from build123d import *

# Parameters (mm, degrees)
SKETCH1_W           = 22.8
SKETCH1_H           = 55
SKETCH1_W_2         = 25
SKETCH1_H_2         = 6
SKETCH1_W_3         = 7.1
SKETCH1_H_3         = 8.35
SKETCH2_R           = 6.05
BOSS_EXTRUDE1_DEPTH = 5.6
SKETCH2_3_W         = 10.7
SKETCH2_3_H         = 16.7
BOSS_EXTRUDE2_DEPTH = 13.8


with BuildPart() as part:
    # Sketch1 → Revolve1 (revolve)
    with BuildSketch(Plane.XY, mode=Mode.PRIVATE) as revolve1_sk:
        with BuildLine():
            Line((-24.6, 0), (0, 0))
            Line((0, 0), (0, 100))
            ThreePointArc((0, 100), (-13.097327972, 97.679363123), (-24.6, 91))
            Line((-24.6, 91), (-24.6, 68.856406461))
            Line((-24.6, 68.856406461), (-24.6, 0))
        make_face()
        with BuildLine():
            Line((0, 100), (0, 0))
            Line((0, 0), (24.6, 0))
            Line((24.6, 0), (24.6, 68.856406461))
            Line((24.6, 68.856406461), (24.6, 91))
            ThreePointArc((24.6, 91), (13.097327972, 97.679363123), (0, 100))
        make_face()
        Polygon((-32.6, 0), (-24.6, 0), (-24.6, 68.856406461), (-32.6, 55), align=None)
        with Locations((-44, 27.5)):
            Rectangle(SKETCH1_W, SKETCH1_H)
        Polygon((-60.4, 0), (-55.4, 0), (-55.4, 11.25), (-60.4, 11.25), (-60.4, 6), align=None)
        with Locations((-72.9, 3)):
            Rectangle(SKETCH1_W_2, SKETCH1_H_2)
        Polygon((24.6, 68.856406461), (24.6, 0), (32.6, 0), (32.6, 26.3), (32.6, 55), align=None)
        Polygon((34.4, 14.85), (34.4, 0), (38.9, 0), (38.9, 8.35), (38.9, 14.85), align=None)
        Polygon((32.6, 26.3), (32.6, 0), (34.4, 0), (34.4, 14.85), (34.4, 26.3), align=None)
        with Locations((42.45, 4.175)):
            Rectangle(SKETCH1_W_3, SKETCH1_H_3)
        with Locations((65.5, 3)):
            Rectangle(SKETCH1_W_2, SKETCH1_H_2)
        Polygon((46, 8.35), (46, 0), (53, 0), (53, 6), (53, 6.65), align=None)
    revolve(revolve1_sk.sketch.rotate(Axis((0, 0, 0), (-1, 0, 0)), 90), axis=Axis((0, 0, 0), (-1, 0, 0)))

    # Sketch2 → Boss-Extrude1 (add)
    with BuildSketch(Plane.ZY.offset(55.4)):
        with Locations((22.627416998, 22.627416998)):
            Circle(SKETCH2_R)
    extrude(amount=BOSS_EXTRUDE1_DEPTH)

    # Sketch2_3 → Boss-Extrude2 (add)
    with BuildSketch(Plane.ZY.offset(55.4)):
        with Locations((22.627416998, -26.372583002)):
            Rectangle(SKETCH2_3_W, SKETCH2_3_H)
    extrude(amount=BOSS_EXTRUDE2_DEPTH)


solid = part.part
Work out the finished part from the listing and answer in its coordinate system (mm). A direction names the side the tool comes from. Give positions to 0.01 mm unless a question says otherwise; leave off trailing zeros. Write each loop counter-clockwise with the first axis right and the second up, starting at its lowest first coordinate (ties: lowest second). Pieces come first, ordered by that corner, then holes. Notation, with made-up numbers: (-28.5, 15) - (18.5, 15) arc R13 cw to (18.5, 22) - close; hole circle Ø3 at (66.25, -33). An arc over 180 degrees is marked (long way). One line per item, written item: value. Start each with the question number.
1. For faces 1 (the flat face through (-24.6, -68, 14)), 2 (the cylindrical face through (42.5, -2.508, -7.964)), 3 (the flat face through (-62, -26, 17.277)), determine the directions among +Z, -Z, +X, -X, +Y, -Y from which every point of the face is accessible in a straight line to the end or side of a thin tool.
2. Find section A-A (x = 61.5). Write down the section's boundary in (y, z), then the cut area to 3 significant figures.
3. Consider probe 1 along X at (y, z) = (46, -24); probe 2 along X at (y, z) = (-43, 61); probe 3 along Y at (x, z) = (-24.5, 5). Determine where each line is inside the solid, lowest interval first.
4. Given pin 1 (6 mm diameter, centred on y = -17.5, z = 65, fed in from -X); pin 2 (4 mm diameter, centred on x = -2.5, z = -14, fed in from -Y); pin 3 (5 mm diameter, centred on x = -44.5, y = -53.5, fed in from +Z), each flat-ended and moving along its own axis, determine where each tip first touches the part or whether it passes through.
5. For a pull along Y with two mould halves and no side action, classify faces 4 (the flat face through (-85.4, 0, 0)), 5 (the flat face through (-62, -34.723, 23)), 6 (the cylindrical face through (33.487, -7.9, -25.086)), 7 (the flat face through (-62, -18.023, 23)) as +Y half, -Y half, draft (parallel to the pull), parting line (faces both ways), or undercut.
6. Find section B-B (x = -16). Write down the section's boundary in (y, z).
Geometry results:
1. face 1: -X
1. face 2: +X
1. face 3: -Z, -X, -Y
2. outline: circle Ø12 at (0, 0)
2. area: 113 mm2
3. probe 1: -55.4 to 32.6
3. probe 2: -24.6 to 24.6
3. probe 3: -90.95 to 90.95
4. pin 1: x = -27.22
4. pin 2: y = -99.22
4. pin 3: z = 20.59
5. face 4: draft
5. face 5: -Y half
5. face 6: parting line
5. face 7: undercut
6. outline: circle Ø192.96 at (0, 0)
